Verification items for the finished model (mm, model axes). Face numbers are marked on the shaded views. A direction names the side the tool comes from. Give positions to 0.01 mm unless a question says otherwise; leave off trailing zeros. Loops run counter-clockwise (first coordinate to the right, second up) from the corner with the lowest first, then second, coordinate; pieces in that order, holes last. Notation, with made-up numbers: M 60.5,85.5 L 92.5,85.5 A14 ccw 92.5,97.5 Z; hole C 39,-12.5 d1. An arc over 180 degrees is marked long. Use a Markdown table: item, result.
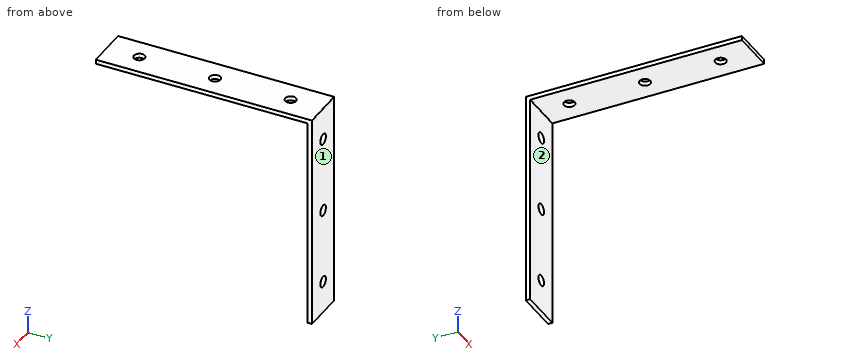
from build123d import *

# Parameters (mm, degrees)
EXTRUSION1_DEPTH = 20
HOLE1_D          = 5
HOLE2_D          = 5


with BuildPart() as part:
    # Sketch1 → Extrusion1 (new body)
    with BuildSketch(Plane.YZ):
        with BuildLine():
            Line((0, -100), (0, -0.2))
            ThreePointArc((0, -0.2), (-0.058578644, -0.058578644), (-0.2, 0))
            Line((-0.2, 0), (-100, 0))
            Line((-100, 0), (-100, -2))
            Line((-100, -2), (-2.2, -2))
            ThreePointArc((-2.2, -2), (-2.058578644, -2.058578644), (-2, -2.2))
            Line((-2, -2.2), (-2, -100))
            Line((-2, -100), (0, -100))
        make_face()
    extrude(amount=EXTRUSION1_DEPTH)

    # Hole1 (through all)
    with Locations(Plane(origin=(0, 0, 0), x_dir=(1, 0, 0), z_dir=(0, 1, 0))):
        with Locations((10, 15), (10, 50), (10, 85)):
            Hole(HOLE1_D / 2)

    # Hole2 (through all)
    with Locations(Plane.XY):
        with Locations((10, -85), (10, -50), (10, -15)):
            Hole(HOLE2_D / 2)


solid = part.part
(1) Cross-section at A-A on x = 10. State how many separate pieces and enclosed holes the cut face has, then the cut area to 3 significant figures.
Results below:
| item | result |
|---|---|
| separate pieces | 7 |
| enclosed holes | 0 |
| area | 336 mm^2 |
(2) Cross-section at D-D on x = 3. Record the cut outline in (y, z), then the cut area to 3 significant figures.
Results below:
| item | result |
|---|---|
| outline | M -100,-2 L -2.2,-2 A0.2 cw -2,-2.2 L -2,-100 L 0,-100 L 0,-0.2 A0.2 ccw -0.2,0 L -100,0 Z |
| area | 396 mm^2 |
(3) Cross-section at B-B on z = -85. Record the cut outline in (x, y).
Results below:
| item | result |
|---|---|
| outline | M 0,-2 L 7.5,-2 L 7.5,0 L 0,0 Z; M 12.5,-2 L 20,-2 L 20,0 L 12.5,0 Z |
(4) Material ranges on line 1 (Z direction, x = 10, y = -0.6); line 2 (X direction, y = -1, z = -15), recorded low to high.
Results below:
| item | result |
|---|---|
| line 1 | -100 to -87.5, -82.5 to -52.5, -47.5 to -17.5, -12.5 to 0 |
| line 2 | 0 to 7.5, 12.5 to 20 |
(5) Gauge pin test, flat ends, axial feed: P1, Ø8, axis at x = 10, y = -50, coming from the -Z side; P2, Ø10, axis at x = 6, z = -27.5, coming from the -Y side. Record the tip position at first contact, or that the pin passes through.
Results below:
| item | result |
|---|---|
| P1 | z = -2 |
| P2 | y = -2 |
(6) Set-up check for the marked faces 1 and 2: record each of +Z, -Z, +X, -X, +Y, -Y from which the full face is reachable in a straight line by a thin tool's end or side.
Results below:
| item | result |
|---|---|
| face 1 | +Z, -Z, +X, -X, +Y |
| face 2 | -Z, +X, -X, -Y |
